Autodesk Inventor part; units mm, degrees
ref_plane "YZ Plane" through (0, 0, 0) normal (1, 0, 0) x (0, 1, 0)
ref_plane "XZ Plane" through (0, 0, 0) normal (0, 1, 0) x (-1, 0, 0)
ref_plane "XY Plane" through (0, 0, 0) normal (0, 0, 1) x (1, 0, 0)
sketch "Sketch1" plane through (0, 0, 0) normal (0, 0, 1) x (1, 0, 0)
  line L0 (0, 0) -> (0, 10)
  line L1 (0, 10) -> (4.6, 10)
  line L2 (4.6, 10) -> (4.6, 2.5)
  line L3 (4.6, 2.5) -> (7.6, 2.5)
  line L4 (7.6, 2.5) -> (7.6, 10)
  line L5 (7.6, 10) -> (12.2, 10)
  line L6 (12.2, 10) -> (12.2, 0)
  line L7 (12.2, 0) -> (0, 0)
  dimension "d0" = 12.2
  dimension "d1" = 10
  dimension "d2" = 7.5
  dimension "d3" = 3
extrude "Extrusion1" add sketch "Sketch1" along normal blind 5
sketch "Sketch2" plane through (0, 0, 0) normal (0, -1, 0) x (1, 0, 0)
  line L0 (0, 0) -> (0, 5)
  line L1 (1.5, 3.77) -> (10.7, 3.77) construction
  line L2 (0, 5) -> (12.2, 5) construction
  line L3 (1.275, 3.995) -> (1.725, 3.995)
  line L4 (1.725, 3.995) -> (1.725, 3.545)
  line L5 (1.725, 3.545) -> (1.275, 3.545)
  line L6 (1.275, 3.545) -> (1.275, 3.995)
  line L7 (1.275, 3.995) -> (1.725, 3.545) construction
  line L8 (1.725, 3.995) -> (1.275, 3.545) construction
  point P0 (1.5, 1.23)
  point P1 (3, 2.5)
  point P2 (10.7, 1.23)
  point P3 (0, 2.5)
  point P4 (6.1, 3.77)
  point P5 (6.1, 5)
  dimension "d6" = 1.27
  dimension "d7" = 1.27
  dimension "d8" = 1.5
  dimension "d9" = 9.2
  dimension "d10" = 0.45
  dimension "d11" = 0.45
extrude "Extrusion2" add sketch "Sketch2" along normal blind 3
pattern_sketch "Sketch Driven Pattern1" of "Extrusion2" from (1.5, 0, 3.77) copies at (1.5, 0, 1.23) at (3, 0, 2.5) at (10.7, 0, 3.77) at (10.7, 0, 1.23)
chamfer "Chamfer1" distance 0.75 angle 45 2 edges at (9.9, 10, 0) (2.3, 10, 0)
properties part number "GP1A52HRJ00F (Large slot detector)"
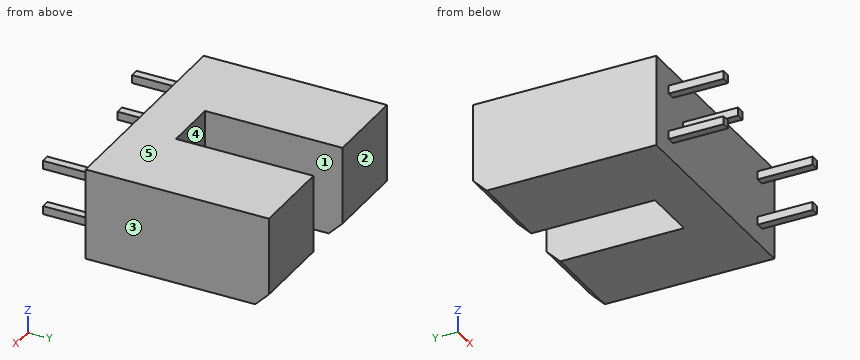
For this review, take the finished solid that the model builds, in its own axes (mm). Face numbers are marked on the shaded views. A direction names the side the tool comes from. Give positions to 0.01 mm unless a question says otherwise; leave off trailing zeros. Write each loop counter-clockwise with the first axis right and the second up, starting at its lowest first coordinate (ties: lowest second). Pieces come first, ordered by that corner, then holes. Notation, with made-up numbers: M -22,76 L 9,76 A17 ccw 9,100 Z; hole C 35,71.25 d4. An arc over 180 degrees is marked long. Answer as a JSON object with one key per item and string values. Group by question number.
Item 1: Tool access review of the marked faces 1 and 2: name each direction out of +Z, -Z, +X, -X, +Y, -Y from which nothing blocks a thin tool from reaching the whole face with its end or side.
Item 2: Draft analysis for pull direction X (two halves, no side actions). For the marked faces 3, 4 and 5, state which applies: +X half, -X half, draft (parallel to the pull), parting line (faces both ways), or undercut.
Item 3: Consider section D-D on x = 8.25. Write out the cut boundary in (y, z), plus the area to 3 significant figures.
Item 4: Consider section B-B on y = 7.5. Write out the cut boundary in (x, z).
Item 5: For pin 1 Ø0.5 at (x, y) = (10.5, -2) entering from -Z (3 decimals); pin 2 Ø0.5 at (x, y) = (3, -2) entering from +Z (3 decimals); pin 3 Ø1 at (x, z) = (8, 3.5) entering from -Y, all flat-tipped, find the tip position at first contact; note any pin that passes through.
Item 6: Consider section A-A on y = -0.5. Write out the cut boundary in (x, z) (3 decimals).
Item 7: Consider section C-C on z = 0.55. Write out the cut boundary in (x, y).
Item 8: For probe 1 along X at (y, z) = (3, 0.5); probe 2 along Y at (x, z) = (6.5, 3.4); probe 3 along Y at (x, z) = (9.5, 2.7), list the stretches that pass through material, from the lowest coordinate up. Write a range as [from, to].
Check result:
{
 "1": {"face 1": "+Z, -Z, +Y", "face 2": "+Z, -Z, +X, -X, +Y"},
 "2": {"face 3": "+X half", "face 4": "undercut", "face 5": "draft"},
 "3": {"outline": "M 0,0 L 9.25,0 L 10,0.75 L 10,5 L 0,5 Z", "area": "49.7 mm^2"},
 "4": {"outline": "M 0,0 L 4.6,0 L 4.6,5 L 0,5 Z; M 7.6,0 L 12.2,0 L 12.2,5 L 7.6,5 Z"},
 "5": {"pin 1": "stops at z = 1.005", "pin 2": "stops at z = 2.725", "pin 3": "stops at y = 0"},
 "6": {"outline": "M 1.275,1.005 L 1.725,1.005 L 1.725,1.455 L 1.275,1.455 Z; M 1.275,3.545 L 1.725,3.545 L 1.725,3.995 L 1.275,3.995 Z; M 2.775,2.275 L 3.225,2.275 L 3.225,2.725 L 2.775,2.725 Z; M 10.475,1.005 L 10.925,1.005 L 10.925,1.455 L 10.475,1.455 Z; M 10.475,3.545 L 10.925,3.545 L 10.925,3.995 L 10.475,3.995 Z"},
 "7": {"outline": "M 0,0 L 12.2,0 L 12.2,9.8 L 7.6,9.8 L 7.6,2.5 L 4.6,2.5 L 4.6,9.8 L 0,9.8 Z"},
 "8": {"probe 1": "x = [0, 4.6], [7.6, 12.2]", "probe 2": "y = [0, 2.5]", "probe 3": "y = [0, 10]"}
}
